CAD build for the part. Positions are in the model's coordinates, mm. A direction names the side the tool comes from. Coordinates: 2 decimals unless noted, no trailing zeros. Write each loop counter-clockwise with the first axis right and the second up, starting at its lowest first coordinate (ties: lowest second). Pieces come first, ordered by that corner, then holes. Notation, with made-up numbers: (19, 20) - (75, 20) arc R16 cw to (75, 43) - close; hole circle Ø9 at (-8.5, -25). An arc over 180 degrees is marked (long way). Answer in a Markdown table with one row per item. Add a question column.
Q1. Band-saw the part on B-B (z = 2.7). List the corners of the cut face in (x, y), and give its area (3 significant figures).
Q2. 3-axis set-ups, long thin cutter, end or side, ignore diameter. For faces 4 (the flat face through (42.948, 0.986, 23.947)), 5 (the flat face through (41.437, 4, 12)), 6 (the flat face through (36, 4, 6.833)), 7 (the flat face through (30.658, 4, 12)), 8 (the flat face through (45.9, 1, 11)): which of +Z, -Z, +X, -X, +Y, -Y reach the whole face in a straight line?
Q3. Pin check, flat tips, straight feed: pin 1 (1 mm diameter, centred on x = 10, z = 3.5, fed in from -Y); pin 2 (1.2 mm diameter, centred on y = 5, z = 10, fed in from +X); pin 3 (3 mm diameter, centred on y = 4, z = 12.5, fed in from -X); pin 4 (8 mm diameter, centred on x = 24, z = 19, fed in from +Y). Stop position of each tip, or through.
Q4. Drill centre lines: line 1 along X through (y, z) = (1, 2.7); line 2 along Y through (x, z) = (28, 2.5); line 3 along Z through (x, y) = (34, 4.35). Where is each one in solid material? Low to high. Write a range as from..to.
Q5. Band-saw the part on A-A (x = 35.4). List the corners of the cut face in (y, z), and give its area (3 significant figures).
Q6. Two-plate mould, pull along X, no slides. Class faces 1 (the flat face through (0, 1, 12)), 2 (the cylindrical face through (34.424, 1.014, 22.608)), 3 (the flat face through (36, 4, 17.644)): +X half, -X half, draft (parallel to the pull), parting line (faces both ways), or undercut.
Q7. Band-saw the part on D-D (z = 11.75). List the corners of the cut face in (x, y).
Q8. Band-saw the part on C-C (y = 1.3). List the corners of the cut face in (x, z), and give its area (3 significant figures).
```python
from build123d import *

# Parameters (mm, degrees)
EXTRUDE_2_DEPTH     = 2
SKETCH_2_W          = 10.779016103
SKETCH_2_H          = 10.811001315
EXTRUDE_3_DEPTH     = 4
SKETCH_3_R          = 1.1
CUT_EXTRUDE_1_DEPTH = 4


with BuildPart() as part:
    # 草图1 → 凸台-拉伸2 (new body)
    with BuildSketch(Plane(origin=(0, 0, 0), x_dir=(1, 0, 0), z_dir=(0, 1, 0))):
        Polygon((0, 0), (45.9, 0), (45.9, -21.658695652), (39.913043478, -26.3), (11.504347826, -26.3), (0, -23.536956522), align=None)
    extrude(amount=EXTRUDE_2_DEPTH)

    # 草图2 → 凸台-拉伸3 (add)
    with BuildSketch(Plane(origin=(0, 2, 0), x_dir=(1, 0, 0), z_dir=(0, 1, 0))):
        with Locations((36.047943901, -12.238421487)):
            Rectangle(SKETCH_2_W, SKETCH_2_H)
    extrude(amount=EXTRUDE_3_DEPTH)

    # 草图3 → 切除-拉伸1 (cut)
    with BuildSketch(Plane(origin=(0, 2, 0), x_dir=(1, 0, 0), z_dir=(0, 1, 0))):
        with Locations(Location((2.7, -2.7, 0), (0, 0, 270))):
            Circle(SKETCH_3_R)
        with Locations(Location((35.4, -22.1, 0), (0, 0, 270))):
            Circle(SKETCH_3_R)
    extrude(amount=-CUT_EXTRUDE_1_DEPTH, mode=Mode.SUBTRACT)


solid = part.part
```
Checked values:
| question | item | result |
|---|---|---|
| 1 | outline | (0, 0) - (1.6, 0) - (1.6, 2) - (0, 2) - close; (3.8, 0) - (45.9, 0) - (45.9, 2) - (3.8, 2) - close |
| 1 | area | 87.4 mm² |
| 2 | face 4 | +Z, +X, +Y, -Y |
| 2 | face 5 | +Z, -Z, +X, +Y |
| 2 | face 6 | -Z, +X, -X, +Y |
| 2 | face 7 | +Z, -Z, -X, +Y |
| 2 | face 8 | +Z, -Z, +X, +Y, -Y |
| 3 | pin 1 | stops at y = 0 |
| 3 | pin 2 | stops at x = 41.44 |
| 3 | pin 3 | stops at x = 30.66 |
| 3 | pin 4 | stops at y = 2 |
| 4 | line 1 | x = 0..1.6, 3.8..45.9 |
| 4 | line 2 | y = 0..2 |
| 4 | line 3 | z = 6.83..17.64 |
| 5 | outline | (0, 0) - (2, 0) - (2, 6.83) - (6, 6.83) - (6, 17.64) - (2, 17.64) - (2, 21) - (0, 21) - close; (0, 23.2) - (2, 23.2) - (2, 26.3) - (0, 26.3) - close |
| 5 | area | 91.4 mm² |
| 6 | face 1 | -X half |
| 6 | face 2 | undercut |
| 6 | face 3 | draft |
| 7 | outline | (0, 0) - (45.9, 0) - (45.9, 2) - (41.44, 2) - (41.44, 6) - (30.66, 6) - (30.66, 2) - (0, 2) - close |
| 8 | outline | (0, 0) - (45.9, 0) - (45.9, 21.66) - (39.91, 26.3) - (11.5, 26.3) - (0, 23.54) - close; hole circle Ø2.2 at (2.7, 2.7); hole circle Ø2.2 at (35.4, 22.1) |
| 8 | area | 1,170 mm² |
